Geometry: final body of the model. Coordinates: model frame, mm. Give positions to 0.01 mm unless a question says otherwise; leave off trailing zeros. Write each loop counter-clockwise with the first axis right and the second up, starting at its lowest first coordinate (ties: lowest second). Pieces come first, ordered by that corner, then holes. Notation, with made-up numbers: (49.5, 11.5) - (54.5, 11.5) arc R30 ccw to (54.5, 45.5) - close; hole circle Ø1 at (45, 31.5). An arc over 180 degrees is marked (long way). Return JSON: item names as keys, results as strings.
from build123d import *

# Parameters (mm, degrees)
F0_R     = 38.1
F0_R_2   = 34.925
F1_DEPTH = 73.025
F2_R     = 38.1
F2_R_2   = 33.3375
F3_DEPTH = 50.8


# Not quite as in the source:
# - a fillet or chamfer that OpenCascade refuses, or shapes differently, is made with other operations: its cross-section is extruded or revolved along the edge and cut away or added


with BuildPart() as f1:
    # F0 (on Top) → F1 (new body)
    with BuildSketch(Plane.XY):
        Circle(F0_R)
        Circle(F0_R_2, mode=Mode.SUBTRACT)
    extrude(amount=F1_DEPTH)

    # F2 (on Top) → F3 (join)
    with BuildSketch(Plane.XY):
        Circle(F2_R)
        Circle(F2_R_2, mode=Mode.SUBTRACT)
    extrude(amount=-F3_DEPTH)

    # F4: fillet of radius 5.08 on 1 edges, made by hand

    # F4_s1 → F4_t2 (revolve, cut)
    with BuildSketch(Plane.XZ):
        with BuildLine():
            ThreePointArc((38.1, 68.3157139607), (37.2321134838, 71.1555202921), (34.925, 73.025))
            Line((34.925, 73.025), (38.1, 73.025))
            Line((38.1, 73.025), (38.1, 68.3157139607))
        make_face()
    revolve(axis=Axis((0, 0, 73.025), (0, 0, 1)), mode=Mode.SUBTRACT)


solid = f1.part
Q1. Section query A-A, the plane y = 0. Return the cut outline in (x, z) (1 decimal), plus the area to 3 significant figures.
Answer key:
{"outline": "(-38.1, -50.8) - (-33.3, -50.8) - (-33.3, 0) - (-34.9, 0) - (-34.9, 73) arc R5.1 ccw to (-38.1, 68.3) - close; (33.3, -50.8) - (38.1, -50.8) - (38.1, 68.3) arc R5.1 ccw to (34.9, 73) - (34.9, 0) - (33.3, 0) - close", "area": "939 mm^2"}
Q2. Material intervals for probe 1 along Y at (x, z) = (0, -13); probe 2 along Y at (x, z) = (0, 43) (3 decimals); probe 3 along Z at (x, y) = (21, 26), sorted ascending. Write a range as [from, to].
Answer key:
{"probe 1": "y = [-38.1, -33.34], [33.34, 38.1]", "probe 2": "y = [-38.1, -34.925], [34.925, 38.1]", "probe 3": "z = [-50.8, 0]"}
Q3. Pin query (flat end, axial travel): P1, Ø1, axis at y = -4.5, z = 32.5, coming from the +X side; P2, Ø1, axis at x = -19, z = 21, coming from the +Y side; P3, Ø8, axis at x = 25, z = 26.5, coming from the +Y side. Return the tip coordinate at first contact, or that it passes through.
Answer key:
{"P1": "stops at x = 37.89", "P2": "stops at y = 33.31", "P3": "stops at y = 31.79"}
Q4. Section query D-D, the plane z = 24. Return the cut outline in (x, y) (3 decimals), plus the area to 3 significant figures.
Answer key:
{"outline": "circle Ø76.2 at (0, 0); hole circle Ø69.85 at (0, 0)", "area": "728 mm^2"}
Q5. Mould query, pull axis Y, two halves, no side actions, for faces 1 (the cylindrical face through (-30.235, -23.183, 9.592)), 2 (the cylindrical face through (31.8, 10.01, -25.04)), 3 (the flat face through (0, -34, -50.8)). Classes: pulls with the +Y half, pulls with the -Y half, needs draft (parallel to the pull), parting line crosses it, or undercut.
Answer key:
{"face 1": "parting line crosses it", "face 2": "undercut", "face 3": "needs draft"}
Q6. Section query C-C, the plane z = -3. Return the cut outline in (x, y) (1 decimal), plus the area to 3 significant figures.
Answer key:
{"outline": "circle Ø76.2 at (0, 0); hole circle Ø66.7 at (0, 0)", "area": "1,070 mm^2"}
